Here's the drawing with two shaded views (mm, measured from the low corner). I have some questions. Coordinates: 2 decimals unless noted, no trailing zeros. Order: outer loops, then holes, each group sorted by start corner. A loop starts at its lowest first (then second) coordinate and runs counter-clockwise, first axis right, second up. Notation, with made-up numbers: (-10.75, 63.25) - (44.25, 63.25) arc R31 ccw to (44.25, 102.25) - close; hole circle Ø1 at (15, -3.75). An arc over 180 degrees is marked (long way). Answer as a JSON object with one key per item and string values. Group by question number.
(1) Imagine slicing it at C-C, the plane x = 30. Write out the boundary of the cut face in (y, z).
(2) Imagine slicing it at A-A, the plane z = 54. Write out the boundary of the cut face in (x, y), and give its area (3 significant figures).
(3) Will these pins go through, and if not, where does the flat tip stop? P1, Ø1, axis at x = 23.5, y = 1.5, coming from the +Z side; P2, Ø0.6, axis at x = 39.5, y = 1, coming from the -Z side; P3, Ø1, axis at y = 0.5, z = 51.5, coming from the +X side.
(4) Imagine slicing it at D-D, the plane x = 57.5. Write out the boundary of the cut face in (y, z).
(5) Imagine slicing it at B-B, the plane y = 1.6. Give the number of separate pieces and of enclosed holes in the cut face, and give its area (3 significant figures).
(6) Please list where these lines run through material, in increasing order: probe 1 along X at (y, z) = (1.3, 30); probe 2 along X at (y, z) = (0.8, 50.5); probe 3 along Z at (x, y) = (14, 1.3).
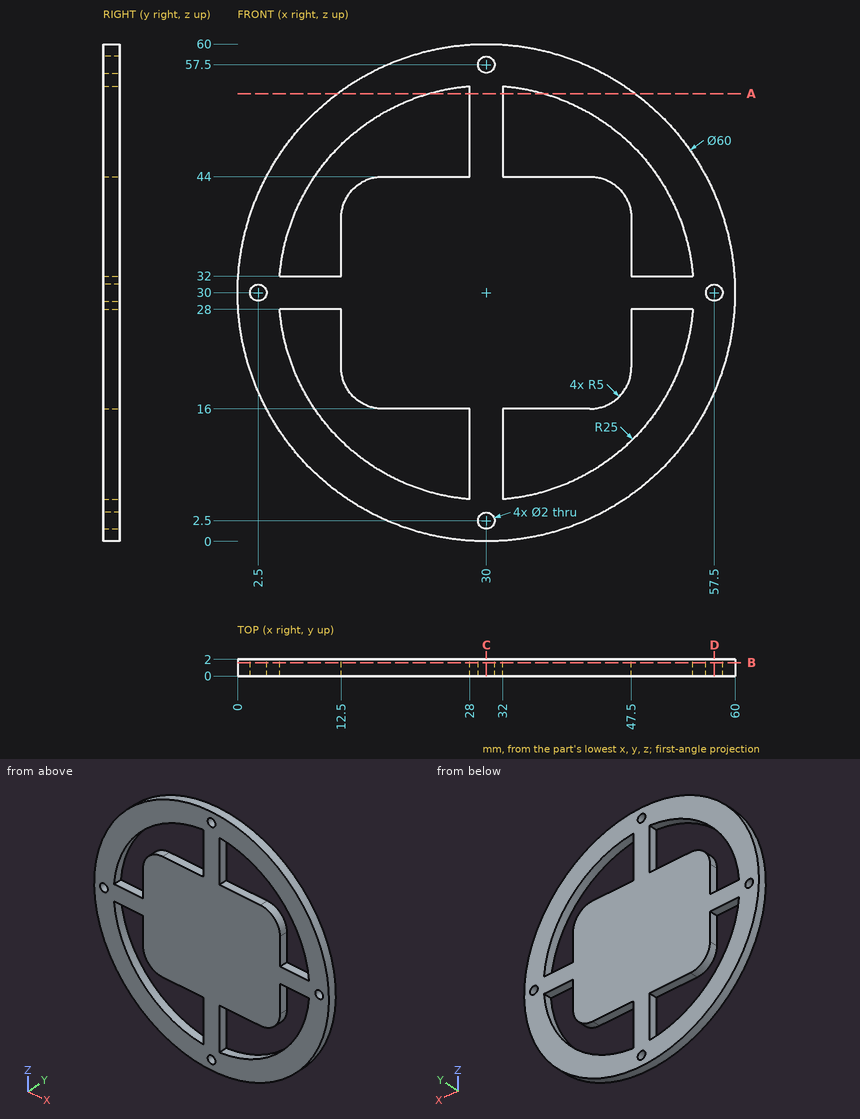
Result set:
{
 "1": {"outline": "(0, 0) - (2, 0) - (2, 1.5) - (0, 1.5) - close; (0, 3.5) - (2, 3.5) - (2, 56.5) - (0, 56.5) - close; (0, 58.5) - (2, 58.5) - (2, 60) - (0, 60) - close"},
 "2": {"outline": "(12, 0) - (23, 0) - (23, 2) - (12, 2) - close; (28, 0) - (32, 0) - (32, 2) - (28, 2) - close; (37, 0) - (48, 0) - (48, 2) - (37, 2) - close", "area": "52.0 mm^2"},
 "3": {"P1": "stops at z = 59.39", "P2": "stops at z = 1.45", "P3": "stops at x = 51.42"},
 "4": {"outline": "(0, 18.01) - (2, 18.01) - (2, 29) - (0, 29) - close; (0, 31) - (2, 31) - (2, 41.99) - (0, 41.99) - close"},
 "5": {"separate pieces": "1", "enclosed holes": "8", "area": "1,960 mm^2"},
 "6": {"probe 1": "x = 0 to 1.5, 3.5 to 56.5, 58.5 to 60", "probe 2": "x = 8.1 to 15.69, 28 to 32, 44.31 to 51.9", "probe 3": "z = 4.62 to 10.79, 17.43 to 42.57, 49.21 to 55.38"}
}
